from build123d import *

# Parameters (mm, degrees)
F0_R     = 18
F1_DEPTH = 5
F2_R     = 15
F3_DEPTH = 5
F4_R     = 5
F5_DEPTH = 10
F6_R     = 5.5
F7_DEPTH = 5
F8_W     = 1.785261
F8_H     = 4
F11_W    = 2.5
F11_H    = 2


with BuildPart() as f1:
    # F0 (on Top) → F1 (new body)
    with BuildSketch(Plane.XY):
        Circle(F0_R)
    extrude(amount=F1_DEPTH)

    # F2 (on face) → F3 (join)
    with BuildSketch(Plane(origin=(0, 0, 0), x_dir=(1, 0, 0), z_dir=(0, 0, -1))):
        Circle(F2_R)
    extrude(amount=F3_DEPTH)

    # F4 (on face) → F5 (cut)
    with BuildSketch(Plane.XY.offset(5)):
        Circle(F4_R)
    extrude(amount=-F5_DEPTH, mode=Mode.SUBTRACT)

    # F6 (on face) → F7 (cut)
    with BuildSketch(Plane.XY.offset(5)):
        Circle(F6_R)
    extrude(amount=-F7_DEPTH, mode=Mode.SUBTRACT)

    # F8 (on Right) → F10 (revolve, cut)
    with BuildSketch(Plane.YZ):
        with Locations((-6.39263, 2)):
            Rectangle(F8_W, F8_H)
    revolve(axis=Axis((0, 0, 2.476329), (0, 0, 1)), mode=Mode.SUBTRACT)

    # F11 (on Right) → F12 (revolve, cut)
    with BuildSketch(Plane.YZ):
        with Locations((6.25, -2.5)):
            Rectangle(F11_W, F11_H)
    revolve(axis=Axis((0, 0, 2.476329), (0, 0, 1)), mode=Mode.SUBTRACT)


solid = f1.part
Here's how the part is built. I have some questions about the finished solid (model axes, mm). A direction names the side the tool comes from. Coordinates: 2 decimals unless noted, no trailing zeros. Write each loop counter-clockwise with the first axis right and the second up, starting at its lowest first coordinate (ties: lowest second). Pieces come first, ordered by that corner, then holes.
1) If we section it at D-D (x = -6): List the corners of the cut face in (y, z) for me.
Filled in:
outline: (-16.97, 0) - (-13.75, 0) - (-13.75, -5) - (13.75, -5) - (13.75, 0) - (16.97, 0) - (16.97, 5) - (-16.97, 5) - close; hole (-4.5, -3.5) - (4.5, -3.5) - (4.5, -1.5) - (-4.5, -1.5) - close; hole (-4.13, 0) - (4.13, 0) - (4.13, 4) - (-4.13, 4) - close
2) If we section it at C-C (z = 1.25): List the corners of the cut face in (x, y) for me.
Filled in:
outline: circle Ø36 at (0, 0); hole circle Ø14.57 at (0, 0)
3) Thinking about a two-plate mould opening in X: for faces 1 (the face through (-4, 15, 0)), 2 (the face through (-1.19, -5.37, 4.51)), 3 (the face through (-14.985, -0.66, -2.465)), which applies, +X half, -X half, draft (parallel to the pull), parting line (faces both ways), or undercut?
Filled in:
face 1: draft
face 2: undercut
face 3: parting line
4) Which directions (+Z, -Z, +X, -X, +Y, -Y) give clear straight access to the entire face, cutting with the end or side of a thin tool? Please do faces 4 (the face through (4.619, -1.915, -4.24)), 5 (the face through (-0.33, -7.493, -2.486)).
Filled in:
face 4: +Z, -Z
face 5: none
5) If I drill on line 1 (Z direction, x = -3, y = -5); line 2 (X direction, y = 0, z = -0.35); line 3 (Y direction, x = 0, z = -2.35), over which ranges is the centre line in solid material (lowest first)?
Filled in:
line 1: z = -5 to -3.5, -1.5 to 0, 4 to 5
line 2: x = -15 to -5, 5 to 15
line 3: y = -15 to -7.5, 7.5 to 15
6) If we section it at A-A (y = 0): List the corners of the cut face in (x, z) for me.
Filled in:
outline: (-18, 0) - (-15, 0) - (-15, -5) - (-5, -5) - (-5, -3.5) - (-7.5, -3.5) - (-7.5, -1.5) - (-5, -1.5) - (-5, 0) - (-7.29, 0) - (-7.29, 4) - (-5.5, 4) - (-5.5, 5) - (-18, 5) - close; (5, -5) - (15, -5) - (15, 0) - (18, 0) - (18, 5) - (5.5, 5) - (5.5, 4) - (7.29, 4) - (7.29, 0) - (5, 0) - (5, -1.5) - (7.5, -1.5) - (7.5, -3.5) - (5, -3.5) - close
7) I'm going to push flat-ended pins straight in: pin 1 (8 mm diameter, centred on x = 0, y = 0, fed in from -Z); pin 2 (1 mm diameter, centred on x = 5, z = 1.5, fed in from +Y); pin 3 (5 mm diameter, centred on x = -7.5, z = 3, fed in from +Y); pin 4 (4.5 mm diameter, centred on x = 3, y = 1, fed in from +Z). Where does each tip first touch, or does it pass through?
Filled in:
pin 1: passes through
pin 2: stops at y = 17.43
pin 3: stops at y = 17.29
pin 4: stops at z = 0
